```python
from build123d import *

# Parameters (mm, degrees)
SKETCH_2_W          = 54
SKETCH_2_H          = 110
EXTRUDE_1_DEPTH     = 5
CUT_EXTRUDE_1_REACH = 64.081
SKETCH_3_R          = 2.4
CHAMFER_1_SIZE      = 1.6


with BuildPart() as part:
    # Эскиз2 → Бобышка-Вытянуть1 (new, symmetric)
    with BuildSketch(Plane(origin=(0, 0, 0), x_dir=(1, 0, 0), z_dir=(0, 1, 0))):
        Rectangle(SKETCH_2_W, SKETCH_2_H)
    extrude(amount=EXTRUDE_1_DEPTH, both=True)

    # Эскиз3 → Вырез-Вытянуть1 (cut, up to next)
    with BuildSketch(Plane(origin=(0, 5, 0), x_dir=(1, 0, 0), z_dir=(0, 1, 0)), mode=Mode.PRIVATE) as cut_extrude_1_sk1:
        with Locations(Location((0, 40, 0), (0, 0, 270))):
            Circle(SKETCH_3_R)
    cut_extrude_1_tool1 = extrude(cut_extrude_1_sk1.sketch, amount=-CUT_EXTRUDE_1_REACH, mode=Mode.PRIVATE) & part.part
    # Эскиз3 → Вырез-Вытянуть1 (cut, up to next)
    with BuildSketch(Plane(origin=(0, 5, 0), x_dir=(1, 0, 0), z_dir=(0, 1, 0)), mode=Mode.PRIVATE) as cut_extrude_1_sk2:
        with Locations(Location((0, -40, 0), (0, 0, 270))):
            Circle(SKETCH_3_R)
    cut_extrude_1_tool2 = extrude(cut_extrude_1_sk2.sketch, amount=-CUT_EXTRUDE_1_REACH, mode=Mode.PRIVATE) & part.part
    add(cut_extrude_1_tool1.solids().sort_by_distance((0, 5, -40))[0], mode=Mode.SUBTRACT)
    add(cut_extrude_1_tool2.solids().sort_by_distance((0, 5, 40))[0], mode=Mode.SUBTRACT)

    # Фаска1
    chamfer_1_edges = [part.edges().sort_by_distance(p)[0] for p in [
        (0, 5, -42.4),
        (0, 5, 37.6),
    ]]
    chamfer(chamfer_1_edges, length=CHAMFER_1_SIZE)


solid = part.part
```
Geometry check sheet. Reference: the model listing, model coordinates, mm. Round coordinates to 2 decimals unless told otherwise and drop trailing zeros. Order: outer loops, then holes, each group sorted by start corner. A loop starts at its lowest first (then second) coordinate and runs counter-clockwise, first axis right, second up. Notation, with made-up numbers: (28, 3) - (84, 3) arc R22 cw to (84, 30) - close; hole circle Ø8 at (-3, -39.75). An arc over 180 degrees is marked (long way). Use a Markdown table: item, result. Add a question column.
(1) Depth check by flat-ended pin: pin 1 (4.5 mm diameter, centred on x = 0, z = -40, fed in from +Y). Enter the tip coordinate at first touch or a pass-through.
(2) Material ranges on line 1 along X through (y, z) = (0.25, -40), recorded low to high. Write a range as [from, to].
(3) Sectioned sample at B-B, the plane z = -40. Enter the section's corners in (x, y).
(4) Release check for a two-part mould opening along X. For faces 1 (the cylindrical face through (0.106, -0.741, -42.398)), 2 (the flat face through (0, 5, -1)), 3 (the flat face through (-27, 0, 1)) record: pulls with the +X half, pulls with the -X half, needs draft (parallel to the pull), parting line crosses it, or undercut.
(5) Sectioned sample at A-A, the plane x = 0. Enter the section's corners in (y, z).
Answers below:
| question | item | result |
|---|---|---|
| 1 | pin 1 | through |
| 2 | line 1 | [-27, -2.4], [2.4, 27] |
| 3 | outline | (-27, -5) - (-2.4, -5) - (-2.4, 3.4) - (-4, 5) - (-27, 5) - close; (2.4, -5) - (27, -5) - (27, 5) - (4, 5) - (2.4, 3.4) - close |
| 4 | face 1 | undercut |
| 4 | face 2 | needs draft |
| 4 | face 3 | pulls with the -X half |
| 5 | outline | (-5, -55) - (5, -55) - (5, -44) - (3.4, -42.4) - (-5, -42.4) - close; (-5, -37.6) - (3.4, -37.6) - (5, -36) - (5, 36) - (3.4, 37.6) - (-5, 37.6) - close; (-5, 42.4) - (3.4, 42.4) - (5, 44) - (5, 55) - (-5, 55) - close |
